Input: part model. Units: mm. Frame: model coordinates. Face numbers are marked on the shaded views. A direction names the side the tool comes from. Coordinates: 2 decimals unless noted, no trailing zeros. Order: outer loops, then holes, each group sorted by start corner. A loop starts at its lowest first (then second) coordinate and runs counter-clockwise, first axis right, second up.
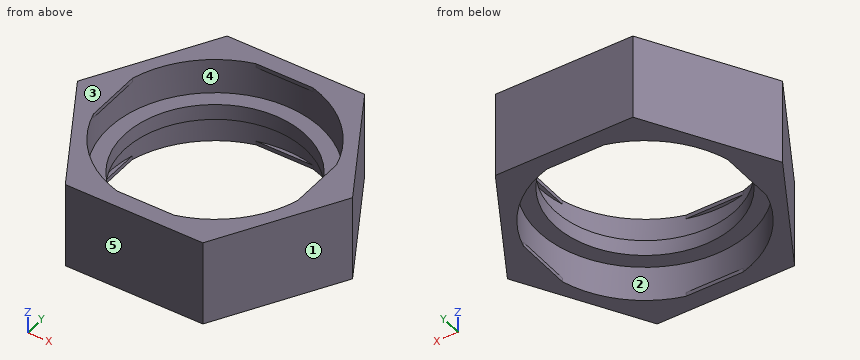
from build123d import *

# Parameters (mm, degrees)
SKETCH001_R      = 40.5
EXTRUDE011_DEPTH = 32.8
EXTRUDE010_DEPTH = 32.8
SKETCH006_R      = 34.5
EXTRUDE009_DEPTH = 6
SKETCH005_R      = 40.5
EXTRUDE008_DEPTH = 6
EXTRUDE005_DEPTH = 1.5
EXTRUDE006_DEPTH = 1.5
EXTRUDE007_DEPTH = 1.5
EXTRUDE004_DEPTH = 1.5
EXTRUDE001_DEPTH = 1.5
EXTRUDE002_DEPTH = 1.5
EXTRUDE003_DEPTH = 1.5
EXTRUDE_DEPTH    = 1.5


with BuildPart() as lid_extrude:
    # Sketch001 (on Sketch) → Extrude011 (new body)
    with BuildSketch(Plane.XY):
        Circle(SKETCH001_R)
    extrude(amount=EXTRUDE011_DEPTH)


with BuildPart() as body:
    # Sketch → Extrude010 (new body)
    with BuildSketch(Plane.XY):
        Polygon((52.540416, 0), (26.270208, 45.501335), (-26.270208, 45.501335), (-52.540416, 0), (-26.270208, -45.501335), (26.270208, -45.501335), align=None)
    extrude(amount=EXTRUDE010_DEPTH)

    # Cut001: cut lid_extrude
    add(lid_extrude.part, mode=Mode.SUBTRACT)


with BuildPart() as lid_divider_in_extrude:
    # Sketch006 → Extrude009 (new body)
    with BuildSketch(Plane.XY):
        Circle(SKETCH006_R)
    extrude(amount=EXTRUDE009_DEPTH)


with BuildPart() as body_divider_fuse:
    # Sketch005 → Extrude008 (new body)
    with BuildSketch(Plane.XY):
        Circle(SKETCH005_R)
    extrude(amount=EXTRUDE008_DEPTH)

    # Cut: cut lid_divider_in_extrude
    add(lid_divider_in_extrude.part, mode=Mode.SUBTRACT)


with BuildPart() as body_divider_fuse_1:
    # Cut placement: moved
    add(body_divider_fuse.part.moved(Location((0, 0, 13.4))))

    # Fusion: union body
    add(body.part)


with BuildPart() as top_teeth1_extrude:
    # MirroredSketch004 → Extrude005 (new body)
    with BuildSketch(Plane.XY):
        with BuildLine():
            Line((10.920165, -39), (-10.920165, -39))
            ThreePointArc((-10.920165, -39), (0, -40.5), (10.920165, -39))
        make_face()
    extrude(amount=EXTRUDE005_DEPTH)


with BuildPart() as top_teeth2_extrude:
    # Sketch007 → Extrude006 (new body)
    with BuildSketch(Plane.XY):
        with BuildLine():
            Line((-39, 10.920165), (-39, -10.920165))
            ThreePointArc((-39, 10.920165), (-40.5, 0), (-39, -10.920165))
        make_face()
    extrude(amount=EXTRUDE006_DEPTH)


with BuildPart() as top_teeth3_extrude:
    # MirroredSketch005 → Extrude007 (new body)
    with BuildSketch(Plane.XY):
        with BuildLine():
            Line((39, -10.920165), (39, 10.920165))
            ThreePointArc((39, -10.920165), (40.5, 0), (39, 10.920165))
        make_face()
    extrude(amount=EXTRUDE007_DEPTH)


with BuildPart() as body_top_teeth_fuse:
    # MirroredSketch003 → Extrude004 (new body)
    with BuildSketch(Plane.XY):
        with BuildLine():
            Line((-10.920165, 39), (10.920165, 39))
            ThreePointArc((10.920165, 39), (0, 40.5), (-10.920165, 39))
        make_face()
    extrude(amount=EXTRUDE004_DEPTH)

    # Compound001: union top_teeth1_extrude, top_teeth2_extrude, top_teeth3_extrude
    add(top_teeth1_extrude.part)
    add(top_teeth2_extrude.part)
    add(top_teeth3_extrude.part)


with BuildPart() as body_top_teeth_fuse_1:
    # Compound001 placement: moved
    add(body_top_teeth_fuse.part.moved(Location((0, 0, 31.3))))

    # Fusion001: union body_divider_fuse
    add(body_divider_fuse_1.part)


with BuildPart() as bottom_teeth1_extrude:
    # MirroredSketch002 → Extrude001 (new body)
    with BuildSketch(Plane.XY):
        with BuildLine():
            Line((-10.920165, 39), (10.920165, 39))
            ThreePointArc((10.920165, 39), (0, 40.5), (-10.920165, 39))
        make_face()
    extrude(amount=EXTRUDE001_DEPTH)


with BuildPart() as bottom_teeth2_extrude:
    # MirroredSketch → Extrude002 (new body)
    with BuildSketch(Plane.XY):
        with BuildLine():
            Line((10.920165, -39), (-10.920165, -39))
            ThreePointArc((-10.920165, -39), (0, -40.5), (10.920165, -39))
        make_face()
    extrude(amount=EXTRUDE002_DEPTH)


with BuildPart() as bottom_teeth3_extrude:
    # Sketch003 → Extrude003 (new body)
    with BuildSketch(Plane.XY):
        with BuildLine():
            Line((-39, 10.920165), (-39, -10.920165))
            ThreePointArc((-39, 10.920165), (-40.5, 0), (-39, -10.920165))
        make_face()
    extrude(amount=EXTRUDE003_DEPTH)


with BuildPart() as body_bottom_teeth_fuse:
    # MirroredSketch001 → Extrude (new body)
    with BuildSketch(Plane.XY):
        with BuildLine():
            Line((39, -10.920165), (39, 10.920165))
            ThreePointArc((39, -10.920165), (40.5, 0), (39, 10.920165))
        make_face()
    extrude(amount=EXTRUDE_DEPTH)

    # Compound: union bottom_teeth1_extrude, bottom_teeth2_extrude, bottom_teeth3_extrude
    add(bottom_teeth1_extrude.part)
    add(bottom_teeth2_extrude.part)
    add(bottom_teeth3_extrude.part)

    # Fusion002: union body_top_teeth_fuse
    add(body_top_teeth_fuse_1.part)


solid = body_bottom_teeth_fuse.part
Item 1: Ray query, probe 1 along Z at (x, y) = (4.5, 39.5); probe 2 along X at (y, z) = (0, 8.75); probe 3 along Y at (x, z) = (0, 7.75). Return the intervals inside material, ascending.
Response values:
probe 1: z = 0 to 1.5, 13.4 to 19.4, 31.3 to 32.8
probe 2: x = -52.54 to -40.5, 40.5 to 52.54
probe 3: y = -45.5 to -40.5, 40.5 to 45.5
Item 2: Cut plane C-C on y = -14. Return loops of the section in (x, z), then the cut area to 3 significant figures.
Response values:
outline: (-44.46, 0) - (-38, 0) - (-38, 13.4) - (-31.53, 13.4) - (-31.53, 19.4) - (-38, 19.4) - (-38, 32.8) - (-44.46, 32.8) - close; (31.53, 13.4) - (38, 13.4) - (38, 0) - (44.46, 0) - (44.46, 32.8) - (38, 32.8) - (38, 19.4) - (31.53, 19.4) - close
area: 501 mm2
Item 3: Draft query along Z for the marked faces 3, 4 and 5. Return one class per face: pulls with the +Z half, pulls with the -Z half, needs draft (parallel to the pull), parting line crosses it, or undercut.
Response values:
face 3: pulls with the +Z half
face 4: undercut
face 5: needs draft
Item 4: Pin query (flat end, axial travel): pin 1 Ø6 at (x, y) = (28, -21.5) entering from +Z; pin 2 Ø3 at (y, z) = (-16.5, 26.5) entering from -X; pin 3 Ø3 at (x, z) = (-30.5, 10.5) entering from +Y. Return the tip coordinate at first contact, or that it passes through.
Response values:
pin 1: stops at z = 19.4
pin 2: stops at x = -43.88
pin 3: stops at y = 40.77
Item 5: Cut plane B-B on z = 27. Return loops of the section in (x, y).
Response values:
outline: (-52.54, 0) - (-26.27, -45.5) - (26.27, -45.5) - (52.54, 0) - (26.27, 45.5) - (-26.27, 45.5) - close; hole circle Ø81 at (0, 0)
Item 6: Cut plane D-D on y = -30.5. Return loops of the section in (x, z), then the cut area to 3 significant figures.
Response values:
outline: (-34.93, 0) - (-26.65, 0) - (-26.65, 13.4) - (-16.12, 13.4) - (-16.12, 19.4) - (-26.65, 19.4) - (-26.65, 32.8) - (-34.93, 32.8) - close; (16.12, 13.4) - (26.65, 13.4) - (26.65, 0) - (34.93, 0) - (34.93, 32.8) - (26.65, 32.8) - (26.65, 19.4) - (16.12, 19.4) - close
area: 670 mm2
Item 7: Access query for the marked faces 1 and 2. Directions: +Z, -Z, +X, -X, +Y, -Y. A direction counts if a zero-diameter tool reaches every point of the face in a straight line with its end or side. Return the directions, or none.
Response values:
face 1: +Z, -Z, +X, -Y
face 2: none
Item 8: Cut plane A-A on x = 0. Return loops of the section in (y, z).
Response values:
outline: (-45.5, 0) - (-39, 0) - (-39, 1.5) - (-40.5, 1.5) - (-40.5, 13.4) - (-34.5, 13.4) - (-34.5, 19.4) - (-40.5, 19.4) - (-40.5, 31.3) - (-39, 31.3) - (-39, 32.8) - (-45.5, 32.8) - close; (34.5, 13.4) - (40.5, 13.4) - (40.5, 1.5) - (39, 1.5) - (39, 0) - (45.5, 0) - (45.5, 32.8) - (39, 32.8) - (39, 31.3) - (40.5, 31.3) - (40.5, 19.4) - (34.5, 19.4) - close
